Here's how the part is built. I have some questions about the finished solid (model axes, mm). Face numbers are marked on the shaded views. A direction names the side the tool comes from. Round coordinates to 2 decimals unless told otherwise and drop trailing zeros. Write each loop counter-clockwise with the first axis right and the second up, starting at its lowest first coordinate (ties: lowest second). Pieces come first, ordered by that corner, then holes. Notation, with made-up numbers: (13, 88.5) - (20, 88.5) arc R19 ccw to (20, 96.5) - close; hole circle Ø5 at (66, -3). An arc over 180 degrees is marked (long way). Write item = value, one per line. Start each with the question number.
Item 1: Which directions (+Z, -Z, +X, -X, +Y, -Y) give clear straight access to the entire face, cutting with the end or side of a thin tool? Please do the marked faces 1 and 2.
Item 2: If I drill on line 1 along Z through (x, y) = (-26, 18); line 2 along Y through (x, z) = (-13, 56.5), over which ranges is the centre line in solid material (lowest first)? Write a range as [from, to].
Item 3: If we section it at C-C (y = 12): Give the number of separate pieces and of enclosed holes in the cut face, and give its area (3 significant figures).
Item 4: For P1, Ø9, axis at y = -3.5, z = 53.5, coming from the -X side; P2, Ø1, axis at x = -50, z = 71, coming from the -Y side; P3, Ø5, axis at x = -19.06, y = 1.74, coming from the +Z side; P4, Ø1.8, axis at x = -19.06, y = 1.74, coming from the -Z side, each with a flat end and sliding along its axis, tell me the tip position at first contact or that it passes through.
Item 5: Thinking about a two-plate mould opening in Z: for the marked faces 3, 4, 5 and 6, which applies, pulls with the +Z half, pulls with the -Z half, needs draft (parallel to the pull), parting line crosses it, or undercut?
Item 6: If we section it at A-A (x = -31): Please give me the cut outline in (y, z).
Item 7: If we section it at B-B (z = 56.5): Please give me the cut outline in (x, y), and give its area (3 significant figures).
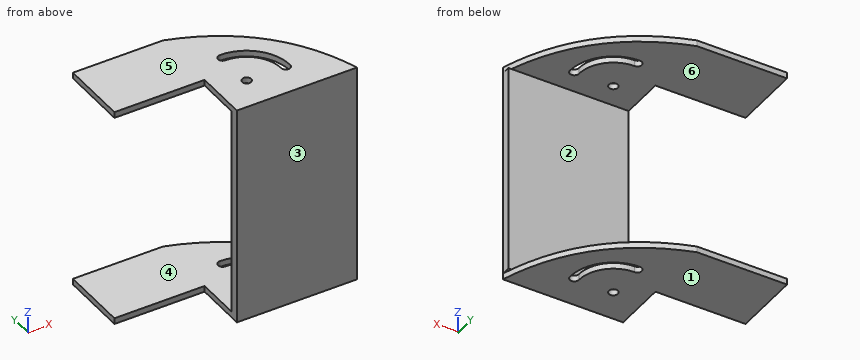
```python
from build123d import *

# Parameters (mm, degrees)
ESQUISSE1_W                = 40
ESQUISSE1_H                = 3
BOSS_EXTRU_2_DEPTH         = 70
ESQUISSE3_R                = 1.5
BOSS_EXTRU_3_DEPTH         = 2
R_P_TITION_LIN_AIRE1_COUNT = 2
R_P_TITION_LIN_AIRE1_PITCH = 72


with BuildPart() as part:
    # Esquisse1 → Boss.-Extru.2 (new body)
    with BuildSketch(Plane.XY):
        with Locations((-9.056759605, -7.756756757)):
            Rectangle(ESQUISSE1_W, ESQUISSE1_H)
    extrude(amount=BOSS_EXTRU_2_DEPTH)

    # Esquisse3 → Boss.-Extru.3 (add)
    with BuildSketch(Plane.XY.offset(70)):
        with BuildLine():
            Line((-29.056759605, -9.256756757), (10.943240395, -9.256756757))
            add(Edge.make_bspline(
                [(-29.056759605, 30.743243243), (1.359242572, 21.353115069), (10.943240395, -9.256756757)],
                knots=[0, 0, 0, 1, 1, 1], degree=2))
            Line((-29.056759605, 30.743243243), (-59.056759605, 30.743243243))
            Line((-59.056759605, 30.743243243), (-59.056759605, 8.243243243))
            Line((-59.056759605, 8.243243243), (-29.056759605, 8.243243243))
            Line((-29.056759605, 8.243243243), (-29.056759605, -9.256756757))
        make_face()
        with Locations((-19.056759605, 1.743243243)):
            Circle(ESQUISSE3_R, mode=Mode.SUBTRACT)
        with BuildLine():
            ThreePointArc((-4.556759605, 1.743243243), (-8.803711277, 11.99629157), (-19.056759605, 16.243243243))
            ThreePointArc((-19.056759605, 16.243243243), (-20.556759605, 14.743243243), (-19.056759605, 13.243243243))
            ThreePointArc((-19.056759605, 13.243243243), (-10.925031621, 9.874971227), (-7.556759605, 1.743243243))
            ThreePointArc((-7.556759605, 1.743243243), (-6.056759605, 0.243243243), (-4.556759605, 1.743243243))
        make_face(mode=Mode.SUBTRACT)
    boss_extru_3 = extrude(amount=BOSS_EXTRU_3_DEPTH)

    # Répétition linéaire1: Boss.-Extru.3 ×2
    with Locations(*[(0, 0, -i * R_P_TITION_LIN_AIRE1_PITCH) for i in range(1, R_P_TITION_LIN_AIRE1_COUNT)]):
        add(boss_extru_3)


solid = part.part
```
Reply:
q1.face_1 = -Z, +X, -X, +Y, -Y
q1.face_2 = +X, -X, +Y
q2.line_1 = [-2, 0], [70, 72]
q2.line_2 = [-9.26, -6.26]
q3.separate_pieces = 4
q3.enclosed_holes = 0
q3.area = 215 mm2
q4.P1 = -29.06
q4.P2 = 8.24
q4.P3 = 72
q4.P4 = through
q5.face_3 = needs draft
q5.face_4 = undercut
q5.face_5 = pulls with the +Z half
q5.face_6 = undercut
q6.outline = (8.24, -2) - (30.74, -2) - (30.74, 0) - (8.24, 0) - close; (8.24, 70) - (30.74, 70) - (30.74, 72) - (8.24, 72) - close
q7.outline = (-29.06, -9.26) - (10.94, -9.26) - (10.94, -6.26) - (-29.06, -6.26) - close
q7.area = 120 mm2
